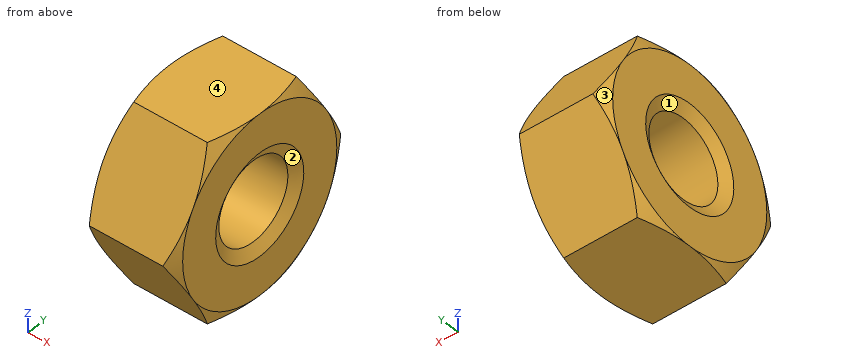
Autodesk Inventor part; units mm, degrees
ref_plane "YZ Plane" through (0, 0, 0) normal (1, 0, 0) x (0, 1, 0)
ref_plane "XZ Plane" through (0, 0, 0) normal (0, 1, 0) x (-1, 0, 0)
ref_plane "XY Plane" through (0, 0, 0) normal (0, 0, 1) x (1, 0, 0)
sketch "Sketch1" plane through (0, 0, 0) normal (1, 0, 0) x (0, 1, 0)
  line L0 (-6.4158, 0) -> (-3.2079, 5.5562)
  line L1 (-3.2079, 5.5562) -> (3.2079, 5.5562)
  line L2 (3.2079, 5.5562) -> (6.4158, 0)
  line L3 (6.4158, 0) -> (3.2079, -5.5562)
  line L4 (3.2079, -5.5562) -> (-3.2079, -5.5563)
  line L5 (-3.2079, -5.5563) -> (-6.4158, 0)
  point P0 (0, 0)
  point P1 (0, 0)
  dimension "d0" = 12.8316
extrude "Body" add sketch "Sketch1" along normal blind 5.5626
sketch "Sketch2" plane through (0, 0, 0) normal (0, 0, 1) x (1, 0, 0)
  line L0 (0, 3.2079) -> (0, 6.4158)
  line L1 (0, 6.4158) -> (5.5626, 6.4158)
  line L2 (5.5626, 3.2079) -> (5.5626, 6.4158)
  line L3 (-0.5563, 0) -> (7.2314, 0)
  line L4 (0.4963, 6.4158) -> (0, 5.5563)
  line L5 (5.0663, 6.4158) -> (5.5626, 5.5563)
  dimension "d3" = 30
  dimension "d4" = 30
  dimension "d5" = 11.1125
  dimension "d6" = 11.1125
revolve "Chamfer1" cut sketch "Sketch2" angle 360 about axis through (-10, 0, 0) along (1, 0, 0)
sketch "Sketch3" plane through (5.5626, 0, 0) normal (1, 0, 0) x (0, 0, -1)
  arc A0 (-2.7781, -4.8119) -> (2.7781, -4.8119) centre (0, 0) ccw
hole "Thread" at (5.5626, 0, 0) direction (-1, 0, 0) diameter 4.9784 end through all
chamfer "Chamfer2" distance 0.6874 angle 30 1 edges at (5.5626, 0, 2.4892) measured on face at (5.5626, 4.5076, -0.1)
chamfer "Chamfer3" distance 0.6874 angle 30 1 edges at (0, 0, 2.4892) measured on face at (0, 4.5076, -0.1)
equation "\"d0\" = 1.1547 * SW"
equation "\"d1\" = KOH"
equation "\"d3\" = ANG1"
equation "\"d4\" = ANG2"
equation "\"d5\" = SW0"
equation "\"d6\" = SW01"
equation "\"d8\" = -0.5 * GD1 + 0.5 * NND"
equation "\"d40\" = -0.5 * GD1 + 0.5 * NND"
equation "\"d10\" = -0.5 * GD1 + 0.5 * NND"
equation "\"d41\" = -0.5 * GD1 + 0.5 * NND"
equation "\"ANG1\" = 30deg"
equation "\"ANG2\" = 30deg"
equation "\"NND\" = 6.35"
equation "\"KOH\" = 5.5626"
equation "\"SW\" = 11.1125"
equation "\"SW0\" = SW"
equation "\"SW01\" = SW"
equation "\"TOA\" = 30deg"
equation "\"THREADDIA\" = 6.35"
equation "\"E0\" = 1.155 * SW"
properties part number "ANSI B18.2.2 - 1/4 - 20" material "Steel, High Strength Low Alloy"
Source: CAD feature listing. Evaluate the final solid. Frame: model axes, mm. Face numbers are marked on the shaded views. Coordinates: 2 decimals unless noted, no trailing zeros. Loops run counter-clockwise (first coordinate to the right, second up) from the corner with the lowest first, then second, coordinate; pieces in that order, holes last. Notation, with made-up numbers: (-38.5, 80) - (-9.5, 80) arc R11 cw to (-9.5, 92) - close; hole circle Ø8 at (-31, 3.25). An arc over 180 degrees is marked (long way). Answer as CSV lines item,"result".
1. Contact query for flat-ended pins moving along their axis: pin 1 (2 mm diameter, centred on x = 3.5, z = -3.5, fed in from +Y); pin 2 (2 mm diameter, centred on x = 1.5, z = 2.5, fed in from -Y); pin 3 (4 mm diameter, centred on y = 0, z = 0, fed in from +X); pin 4 (3 mm diameter, centred on x = 3, z = -2.5, fed in from -Y). Output: stop coordinate, or through.
Established:
pin 1,"stops at y = 4.97"
pin 2,"stops at y = -5.55"
pin 3,"passes through"
pin 4,"stops at y = -5.84"
2. Ray query, line 1 (Z direction, x = 4.1, y = 0); line 2 (Z direction, x = 5.1, y = -0.5); line 3 (Y direction, x = 4.4, z = 2). Return the intervals inside material, ascending.
Established:
line 1,"z = -5.56 to -2.49, 2.49 to 5.56"
line 2,"z = -5.56 to -2.44, 2.44 to 5.56"
line 3,"y = -5.26 to -1.48, 1.48 to 5.26"
3. Mould query, pull axis Z, two halves, no side actions, for the marked faces 1, 2, 3 and 4. Classes: released by +Z, released by -Z, zero draft, split by the parting line, or undercut.
Established:
face 1,"undercut"
face 2,"undercut"
face 3,"split by the parting line"
face 4,"released by +Z"
4. Section A-A (x = 3.7). Return loops of the section in (y, z), then the cut area to 3 significant figures.
Established:
outline,"(-6.42, 0) - (-3.21, -5.56) - (3.21, -5.56) - (6.42, 0) - (3.21, 5.56) - (-3.21, 5.56) - close; hole circle Ø4.98 at (0, 0)"
area,"87.5 mm2"
